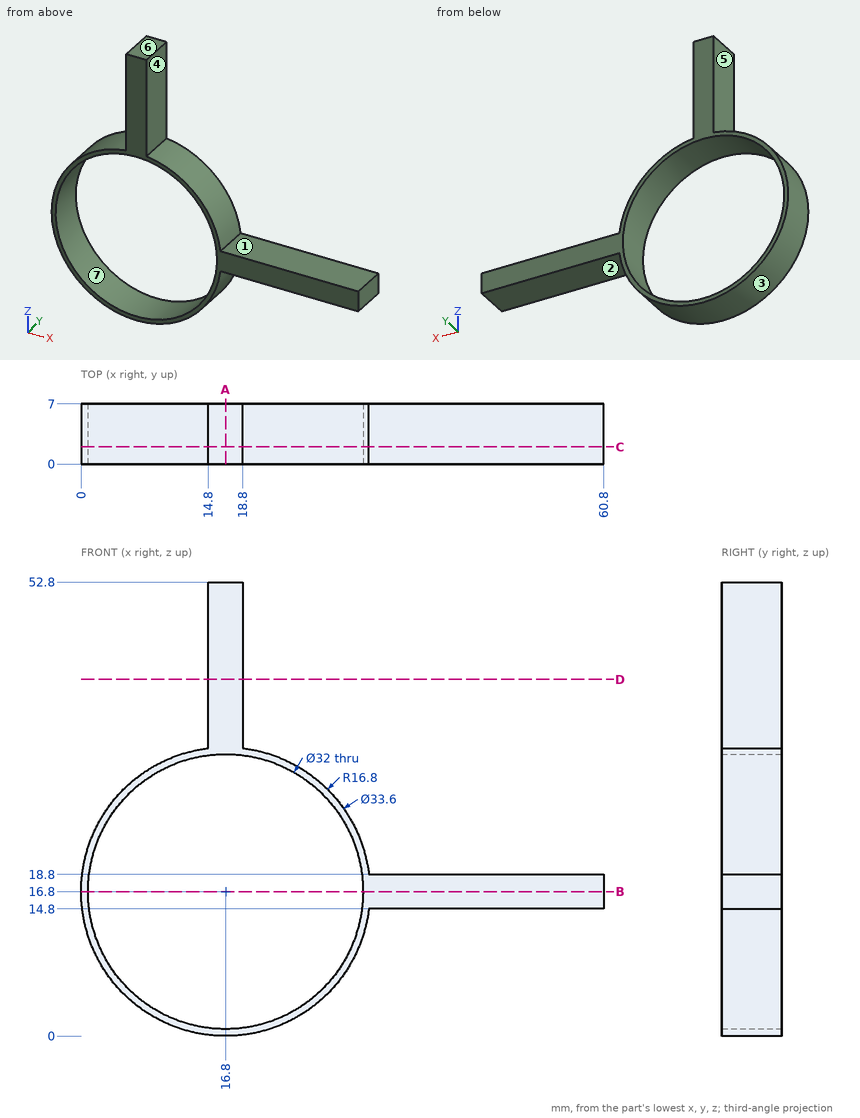
Input: dimensioned drawing with shaded views. Units: mm. Origin: part minimum x, y, z. A direction names the side the tool comes from. Give positions to 0.01 mm unless a question says otherwise; leave off trailing zeros. Order: outer loops, then holes, each group sorted by start corner. A loop starts at its lowest first (then second) coordinate and runs counter-clockwise, first axis right, second up. Notation, with made-up numbers: (56, -23) -> (67, -23) arc R24 cw to (67, 11) -> close; hole circle Ø3 at (80, -35). An arc over 180 degrees is marked (long way). Write item = value, one per line.
Item 1: Set-up query: the marked faces 1, 2 and 3. Return all of +Z, -Z, +X, -X, +Y, -Y with unobstructed straight access to the full face (end or side cutting, diameter ignored); none if empty.
Check result:
face_1 = +Z, +X, +Y, -Y
face_2 = -Z, +X, +Y, -Y
face_3 = +Y, -Y
Item 2: Section query C-C (y = 2). Output: boundary loops of the cut face in (x, z), then the cut area to 3 significant figures.
Check result:
outline = (14.8, 33.48) arc R16.8 ccw (long way) to (33.48, 14.8) -> (60.8, 14.8) -> (60.8, 18.8) -> (33.48, 18.8) arc R16.8 ccw to (18.8, 33.48) -> (18.8, 52.8) -> (14.8, 52.8) -> close; hole circle Ø32 at (16.8, 16.8)
area = 268 mm²
Item 3: Ray query, probe 1 along X at (y, z) = (1.75, 16.8); probe 2 along Z at (x, y) = (51.5, 4); probe 3 along Z at (x, y) = (11.5, 2.25). Return the intervals inside material, ascending.
Check result:
probe_1 = 0 to 0.8, 32.8 to 60.8
probe_2 = 14.8 to 18.8
probe_3 = 0.86 to 1.7, 31.9 to 32.74
Item 4: Section query D-D (z = 41.5). Output: boundary loops of the cut face in (x, y).
Check result:
outline = (14.8, 0) -> (18.8, 0) -> (18.8, 7) -> (14.8, 7) -> close
Item 5: Mould query, pull axis X, two halves, no side actions, for the marked faces 4, 5, 6 and 7. Classes: +X half, -X half, draft (parallel to the pull), parting line (faces both ways), or undercut.
Check result:
face_4 = +X half
face_5 = -X half
face_6 = draft
face_7 = undercut
Item 6: Section query A-A (x = 16.8). Output: boundary loops of the cut face in (y, z), then the cut area to 3 significant figures.
Check result:
outline = (0, 0) -> (7, 0) -> (7, 0.8) -> (0, 0.8) -> close; (0, 32.8) -> (7, 32.8) -> (7, 52.8) -> (0, 52.8) -> close
area = 146 mm²
Item 7: Contact query for flat-ended pins moving along their axis: pin 1 (2 mm diameter, centred on x = 43, y = 2, fed in from +Z); pin 2 (3.5 mm diameter, centred on y = 3.5, z = 45.5, fed in from -X). Output: stop coordinate, or through.
Check result:
pin_1 = 18.8
pin_2 = 14.8
Item 8: Section query B-B (z = 16.8). Output: boundary loops of the cut face in (x, y), then the cut area to 3 significant figures.
Check result:
outline = (0, 0) -> (0.8, 0) -> (0.8, 7) -> (0, 7) -> close; (32.8, 0) -> (60.8, 0) -> (60.8, 7) -> (32.8, 7) -> close
area = 202 mm²
